from build123d import *

# Parameters (mm, degrees)
SKETCH_1_W          = 256
SKETCH_1_H          = 256
EXTRUDE_1_DEPTH     = 100
SKETCH_2_R          = 5
CUT_EXTRUDE_1_DEPTH = 257
CHAMFER_1_SIZE      = 10


with BuildPart() as part:
    # 草圖1 → 填料-伸長1 (new body)
    with BuildSketch(Plane.XY):
        Rectangle(SKETCH_1_W, SKETCH_1_H)
    extrude(amount=EXTRUDE_1_DEPTH)

    # 草圖2 → 除料-伸長1 (cut, through all)
    with BuildSketch(Plane.XZ.offset(128)):
        with Locations((98, 16)):
            Circle(SKETCH_2_R)
    extrude(amount=-CUT_EXTRUDE_1_DEPTH, mode=Mode.SUBTRACT)

    # 導角1
    chamfer_1_edges = [part.edges().sort_by_distance(p)[0] for p in [
        (-128, 0, 100),
        (0, -128, 100),
        (128, 0, 100),
        (0, -128, 0),
        (-128, 0, 0),
        (0, 128, 0),
        (128, 0, 0),
        (0, 128, 100),
    ]]
    chamfer(chamfer_1_edges, length=CHAMFER_1_SIZE)


solid = part.part
Can you work these out from the model? Positions are in its coordinate system, mm. Give positions to 0.01 mm unless a question says otherwise; leave off trailing zeros. Write each loop counter-clockwise with the first axis right and the second up, starting at its lowest first coordinate (ties: lowest second). Pieces come first, ordered by that corner, then holes. Notation, with made-up numbers: (9, 67) -> (34, 67) arc R22 ccw to (34, 87) -> close; hole circle Ø2 at (53, -6). An arc over 180 degrees is marked (long way). Answer as a JSON object with one key per item and string values. Group by question number.
Item 1: Suppose I cut it at A-A (x = 98). Please give me the cut outline in (y, z).
Item 2: Suppose I cut it at B-B (z = 16). Please give me the cut outline in (x, y).
Item 3: Please list where these lines run through material, in increasing order: line 1 (Z direction, x = 98, y = 31); line 2 (Y direction, x = 52, z = 5); line 3 (Y direction, x = -108, z = 90.5). Write a range as [from, to].
Item 4: We'd pull the mould along Z, two halves only. Please class faces 1 (the face through (-2, -123, 5)), 2 (the face through (128, -2, 49)), 3 (the face through (102.619, -1.792, 14.085)): +Z half, -Z half, draft (parallel to the pull), parting line (faces both ways), or undercut.
Findings:
{
 "1": {"outline": "(-128, 10) -> (-118, 0) -> (118, 0) -> (128, 10) -> (128, 11) -> (-128, 11) -> close; (-128, 21) -> (128, 21) -> (128, 90) -> (118, 100) -> (-118, 100) -> (-128, 90) -> close"},
 "2": {"outline": "(-128, -128) -> (93, -128) -> (93, 128) -> (-128, 128) -> close; (103, -128) -> (128, -128) -> (128, 128) -> (103, 128) -> close"},
 "3": {"line 1": "z = [0, 11], [21, 100]", "line 2": "y = [-123, 123]", "line 3": "y = [-127.5, 127.5]"},
 "4": {"face 1": "-Z half", "face 2": "draft", "face 3": "undercut"}
}
